Design review of the part built by this model. Coordinates are the model's own, in mm. Coordinates: 2 decimals unless noted, no trailing zeros. Loops run counter-clockwise (first coordinate to the right, second up) from the corner with the lowest first, then second, coordinate; pieces in that order, holes last. Notation, with made-up numbers: (-38.75, 56) -> (-25.75, 56) arc R20 cw to (-25.75, 72) -> close; hole circle Ø10 at (-19, -25). An arc over 180 degrees is marked (long way). One line per item, written item: value. Start each with the question number.
1. Add section B-B on x = -22.5. Write out the cut boundary in (y, z).
2. Add section C-C on x = 10. Write out the cut boundary in (y, z).
3. Add section D-D on z = -20. Write out the cut boundary in (x, y), plus the area to 3 significant figures.
4. For probe 1 along Z at (x, y) = (11.5, 1); probe 2 along Z at (x, y) = (14.5, 1.1); probe 3 along X at (y, z) = (1.1, -15.25), list the stretches that pass through material, from the lowest coordinate up.
5. Insertion check: pin 1 (1.5 mm diameter, centred on x = 20, y = 1, fed in from -Z); pin 2 (1.5 mm diameter, centred on x = 11.5, y = 2.5, fed in from -Z). Each pin has a flat end and moves straight along its axis. Give the tip position at first contact, or say it passes through.
6. Add section A-A on z = -10. Write out the cut boundary in (x, y).
Autodesk Inventor part; units mm, degrees
ref_plane "YZ Plane" through (0, 0, 0) normal (1, 0, 0) x (0, 1, 0)
ref_plane "XZ Plane" through (0, 0, 0) normal (0, 1, 0) x (-1, 0, 0)
ref_plane "XY Plane" through (0, 0, 0) normal (0, 0, 1) x (1, 0, 0)
sketch "Sketch1" plane through (0, 0, 0) normal (0, 1, 0) x (-1, 0, 0)
  arc A0 (-2.9502, -0.8481) -> (-2.9502, 0.8481) centre (-3.48, 0) ccw
  line L0 (-2.9502, 0.8481) -> (-7.8639, 3.9177)
  arc A1 (-7.8639, 3.9177) -> (-9.3575, 3.336) centre (-8.3937, 3.0696) ccw
  line L1 (-9.3575, 3.336) -> (-10.206, 0.2664)
  arc A2 (-10.206, 0.2664) -> (-10.206, -0.2664) centre (-9.2421, 0) ccw
  line L2 (-10.206, -0.2664) -> (-9.3575, -3.336)
  arc A3 (-9.3575, -3.336) -> (-7.8639, -3.9177) centre (-8.3937, -3.0696) ccw
  line L3 (-7.8639, -3.9177) -> (-2.9502, -0.8481)
  line L4 (-21.4137, 36.6803) -> (-21.3554, 36.5991)
  line L5 (18.0989, 21.6995) -> (22.3004, 27.5465)
  circle A4 centre (27.5044, 32.3038) radius 1.475
  line L6 (7.8639, 3.9177) -> (2.9502, 0.8481)
  arc A5 (2.9502, 0.8481) -> (2.9502, -0.8481) centre (3.48, 0) ccw
  line L7 (2.9502, -0.8481) -> (7.8639, -3.9177)
  arc A6 (7.8639, -3.9177) -> (9.3575, -3.336) centre (8.3937, -3.0696) ccw
  line L8 (9.3575, -3.336) -> (10.206, -0.2664)
  arc A7 (10.206, -0.2664) -> (10.206, 0.2664) centre (9.2421, 0) ccw
  line L9 (10.206, 0.2664) -> (9.3575, 3.336)
  arc A8 (9.3575, 3.336) -> (7.8639, 3.9177) centre (8.3937, 3.0696) ccw
  line L10 (-24.6555, 25.8542) -> (-20.454, 20.0072)
  arc A9 (-20.454, 20.0072) -> (-18.0989, 21.6995) centre (-19.2764, 20.8534) ccw
  line L11 (-18.0989, 21.6995) -> (-22.3004, 27.5465)
  arc A10 (-22.3004, 27.5465) -> (-24.6555, 25.8542) centre (-23.4779, 26.7004) ccw
  line L12 (14.2256, 26.6769) -> (21.4137, 36.6803)
  arc A11 (-26.3995, -17.9136) -> (-26.3995, 17.9136) centre (-51.8984, 0) ccw
  arc A12 (26.3995, 17.9136) -> (26.3995, -17.9136) centre (51.8984, 0) ccw
  line L13 (-21.3365, 36.5729) -> (-12.8954, 24.8295)
  arc A13 (-12.8954, 24.8295) -> (14.2256, 26.6769) centre (-0.0002, 35.5195) ccw
  arc A14 (18.0989, 21.6995) -> (20.454, 20.0072) centre (19.2764, 20.8534) ccw
  line L14 (24.6555, 25.8542) -> (20.454, 20.0072)
  circle A15 centre (15.2498, 15.25) radius 1.475
  arc A16 (-21.3554, 36.5991) -> (-21.3365, 36.5729) centre (0, 51.9445) ccw
  circle A17 centre (-15.2502, 15.25) radius 1.475
  line L15 (33.595, 27.9272) -> (26.3995, 17.9136)
  arc A18 (24.6555, 25.8542) -> (22.3004, 27.5465) centre (23.4779, 26.7004) ccw
  arc A19 (33.595, 27.9272) -> (21.4137, 36.6803) centre (27.5044, 32.3038) ccw
  line L16 (-22.3004, -27.5465) -> (-18.0989, -21.6995)
  arc A20 (-18.0989, -21.6995) -> (-20.454, -20.0072) centre (-19.2764, -20.8534) ccw
  line L17 (-20.454, -20.0072) -> (-24.6555, -25.8542)
  arc A21 (-24.6555, -25.8542) -> (-22.3004, -27.5465) centre (-23.4779, -26.7004) ccw
  circle A22 centre (10, 10) radius 2.1
  circle A23 centre (-10, 10) radius 2.1
  arc A24 (-21.4137, 36.6803) -> (-33.595, 27.9272) centre (-27.5044, 32.3038) ccw
  line L18 (-26.3995, 17.9136) -> (-33.595, 27.9272)
  circle A25 centre (-27.5044, 32.3038) radius 1.475
  line L19 (-21.3554, -36.5991) -> (-21.4137, -36.6803)
  circle A26 centre (15.2498, -15.25) radius 1.475
  line L20 (18.0989, -21.6995) -> (22.3004, -27.5465)
  arc A27 (22.3004, -27.5465) -> (24.6555, -25.8542) centre (23.4779, -26.7004) ccw
  line L21 (24.6555, -25.8542) -> (20.454, -20.0072)
  arc A28 (20.454, -20.0072) -> (18.0989, -21.6995) centre (19.2764, -20.8534) ccw
  circle A29 centre (27.5044, -32.3038) radius 1.475
  circle A30 centre (-10.0002, -10) radius 2.1
  circle A31 centre (10, -10) radius 2.1
  line L22 (-14.2191, -26.666) -> (-21.3554, -36.5991)
  line L23 (21.3554, -36.5991) -> (14.2318, -26.6869)
  circle A32 centre (-15.2502, -15.25) radius 1.475
  circle A33 centre (-27.5044, -32.3038) radius 1.475
  arc A34 (21.4137, -36.6803) -> (33.595, -27.9272) centre (27.5044, -32.3038) ccw
  line L24 (-33.595, -27.9272) -> (-26.3995, -17.9136)
  arc A35 (14.2318, -26.6869) -> (-14.2191, -26.666) centre (-0.0002, -35.5195) ccw
  line L25 (26.3995, -17.9136) -> (33.595, -27.9272)
  line L26 (21.4137, -36.6803) -> (21.3554, -36.5991)
  arc A36 (-33.595, -27.9272) -> (-21.4137, -36.6803) centre (-27.5044, -32.3038) ccw
  line L27 (3.48, 0) -> (-3.48, 0) construction
  point P0 (0, 0)
  point P1 (0, 0)
  point P2 (-21.4137, 36.6803)
  point P3 (-33.595, 27.9272)
  point P4 (-21.4137, -36.6803)
  point P5 (21.4137, -36.6803)
  point P6 (21.4137, 36.6803)
  point P7 (-12.8954, 24.8295)
  point P8 (-21.3365, 36.5729)
  point P9 (-21.3554, 36.5991)
extrude "Extrusion1" add sketch "Sketch1" along normal blind 3 contours L3 A3 L2 A2 L1 A1 L0 A0 | L4 A16 L13 A13 L12 A19 L15 A12 L25 A34 L26 L23 A35 L22 L19 A36 L24 A11 L18 A24 | L5 A18 L14 A14 | A8 L9 A7 L8 A6 L7 A5 L6 | A10 L11 A9 L10 | A21 L17 A20 L16 | A28 L21 A27 L20
sketch "Sketch2" plane through (0, 3, 0) normal (0, 1, 0) x (1, 0, 0)
  circle A0 centre (-15.2498, 15.25) radius 1.475 construction
  circle A1 centre (15.2502, 15.25) radius 1.475 construction
  circle A2 centre (15.2502, -15.25) radius 1.475 construction
  circle A3 centre (-15.2498, -15.25) radius 1.475 construction
  circle A4 centre (-15.2498, 15.25) radius 1.475
  circle A5 centre (-15.2498, 15.25) radius 1.55
  circle A6 centre (15.2502, 15.25) radius 1.475
  circle A7 centre (15.2502, 15.25) radius 1.55
  circle A8 centre (15.2502, -15.25) radius 1.475
  circle A9 centre (15.2502, -15.25) radius 1.55
  circle A10 centre (-15.2498, -15.25) radius 1.55
  point P0 (0, 0)
  dimension "d2" = 3.1
  dimension "d3" = 3.1
  dimension "d4" = 3.1
  dimension "d5" = 3.1
extrude "Extrusion2" cut sketch "Sketch2" against normal through all contours A4 | A5 | A6 | A7 | A8 | A9 | A10
properties part number "bottom plate"
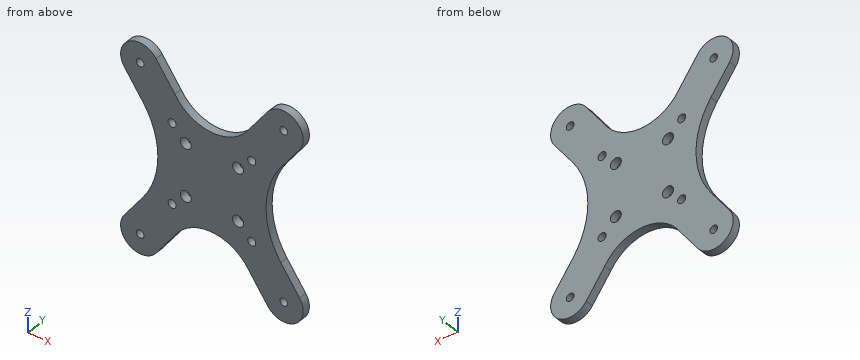
Worked answers:
1. outline: (0, -37.89) -> (3, -37.89) -> (3, -10.34) -> (0, -10.34) -> close; (0, 10.34) -> (3, 10.34) -> (3, 37.89) -> (0, 37.89) -> close
2. outline: (0, -22.08) -> (3, -22.08) -> (3, -12.1) -> (0, -12.1) -> close; (0, -7.9) -> (3, -7.9) -> (3, 7.9) -> (0, 7.9) -> close; (0, 12.1) -> (3, 12.1) -> (3, 22.08) -> (0, 22.08) -> close
3. outline: (-27.9, 0) -> (-6.3, 0) -> (-6.3, 3) -> (-27.9, 3) -> close; (6.3, 0) -> (27.9, 0) -> (27.9, 3) -> (6.3, 3) -> close
3. area: 130 mm²
4. probe 1: z = -23.34 to -11.47, -8.53 to 8.53, 11.47 to 23.34
4. probe 2: z = -27.06 to -16.61, -13.89 to 13.89, 16.61 to 27.06
4. probe 3: x = -24.72 to -16.8, -13.7 to 13.7, 16.8 to 24.72
5. pin 1: stops at z = -35.76
5. pin 2: stops at z = -24.1
6. outline: (-22.38, 0) -> (-12.1, 0) -> (-12.1, 3) -> (-22.38, 3) -> close; (-7.9, 0) -> (7.9, 0) -> (7.9, 3) -> (-7.9, 3) -> close; (12.1, 0) -> (22.38, 0) -> (22.38, 3) -> (12.1, 3) -> close
